from build123d import *

# Parameters (mm, degrees)
SKETCH1_R           = 15.875
SKETCH1_R_2         = 1.5875
BOSS_EXTRUDE1_DEPTH = 6.35
BOSS_EXTRUDE2_START = -6.35
SKETCH2_R           = 1.5875
BOSS_EXTRUDE2_DEPTH = 6.35


with BuildPart() as part:
    # Sketch1 → Boss-Extrude1 (new body)
    with BuildSketch(Plane.XY):
        with BuildLine():
            Line((0, -31.75), (76.2, -31.75))
            Line((76.2, -31.75), (76.2, -6.35))
            Line((76.2, -6.35), (31.108519733, -6.35))
            ThreePointArc((31.108519733, -6.35), (-20.080463142, 24.593444248), (0, -31.75))
        make_face()
        Circle(SKETCH1_R, mode=Mode.SUBTRACT)
        with Locations((-25.4, 0)):
            Circle(SKETCH1_R_2, mode=Mode.SUBTRACT)
        with Locations((25.4, 0)):
            Circle(SKETCH1_R_2, mode=Mode.SUBTRACT)
        with Locations((38.1, -19.05)):
            Circle(SKETCH1_R_2, mode=Mode.SUBTRACT)
        with Locations((63.5, -19.05)):
            Circle(SKETCH1_R_2, mode=Mode.SUBTRACT)
    extrude(amount=BOSS_EXTRUDE1_DEPTH)

    # Sketch2 → Boss-Extrude2 (add)
    with BuildSketch(Plane.XY.offset(6.35).offset(BOSS_EXTRUDE2_START)):
        with BuildLine():
            Line((76.2, -6.35), (76.2, 19.05))
            Line((76.2, 19.05), (25.4, 19.05))
            ThreePointArc((25.4, 19.05), (30.977301377, 6.961989614), (31.108519733, -6.35))
            Line((31.108519733, -6.35), (76.2, -6.35))
        make_face()
        with Locations((63.5, 6.35)):
            Circle(SKETCH2_R, mode=Mode.SUBTRACT)
    extrude(amount=BOSS_EXTRUDE2_DEPTH)


solid = part.part
Work out the finished part from the listing and answer in its coordinate system (mm). A direction names the side the tool comes from. Give positions to 0.01 mm unless a question says otherwise; leave off trailing zeros. Loops run counter-clockwise (first coordinate to the right, second up) from the corner with the lowest first, then second, coordinate; pieces in that order, holes last. Notation, with made-up numbers: (17.5, 45) - (38.5, 45) arc R10 ccw to (38.5, 50) - close; hole circle Ø7 at (80.5, 19.25). An arc over 180 degrees is marked (long way). Answer in a Markdown table with one row per item.
(1) For a pull along Y with two mould halves and no side action, classify faces 1 (the face through (-26.986, 0.07, 3.131)), 2 (the face through (38, -31.75, 3)), 3 (the face through (64.35, -17.71, 3.13)), 4 (the face through (76.2, -7, 3)) as pulls with the +Y half, pulls with the -Y half, needs draft (parallel to the pull), parting line crosses it, or undercut.
Results list:
| item | result |
|---|---|
| face 1 | undercut |
| face 2 | pulls with the -Y half |
| face 3 | undercut |
| face 4 | needs draft |
(2) Section A-A (x = 38.1) is taken. Give the vertices of the cut face in (y, z).
Results list:
| item | result |
|---|---|
| outline | (-31.75, 0) - (-20.64, 0) - (-20.64, 6.35) - (-31.75, 6.35) - close; (-17.46, 0) - (19.05, 0) - (19.05, 6.35) - (-17.46, 6.35) - close |
(3) Flat-ended cylindrical pins translate along their axes: pin 1 Ø8 at (x, y) = (24.5, 5.5) entering from -Z; pin 2 Ø1.9 at (x, y) = (25.4, 0) entering from -Z; pin 3 Ø2 at (y, z) = (-6.5, 2) entering from -X; pin 4 Ø3 at (x, z) = (-20, 4) entering from +Y. Find the tip coordinate at first contact, or state that the pin passes through.
Results list:
| item | result |
|---|---|
| pin 1 | stops at z = 0 |
| pin 2 | passes through |
| pin 3 | stops at x = -31.27 |
| pin 4 | stops at y = 25.8 |
(4) A tool of negligible diameter and unlimited length cuts with its end or side. For faces 5 (the face through (51, 19.05, 3)), 6 (the face through (26.914, 0.477, 3.131)), from which of +Z, -Z, +X, -X, +Y, -Y can it reach the whole face along a straight path? Write none if from no direction.
Results list:
| item | result |
|---|---|
| face 5 | +Z, -Z, +X, +Y |
| face 6 | +Z, -Z |
(5) Section D-D (x = 63.5) is taken. Give the vertices of the cut face in (y, z), and give its area (3 significant figures).
Results list:
| item | result |
|---|---|
| outline | (-31.75, 0) - (-20.64, 0) - (-20.64, 6.35) - (-31.75, 6.35) - close; (-17.46, 0) - (4.76, 0) - (4.76, 6.35) - (-17.46, 6.35) - close; (7.94, 0) - (19.05, 0) - (19.05, 6.35) - (7.94, 6.35) - close |
| area | 282 mm² |
(6) Consider L1, parallel to Y at x = 63.5, z = 4.75; L2, parallel to Y at x = 0, z = 2.25 (3 decimals); L3, parallel to X at y = -1, z = 5.75. Determine where each line is inside the solid, lowest interval first. Write a range as [from, to].
Results list:
| item | result |
|---|---|
| L1 | y = [-31.75, -20.64], [-17.46, 4.76], [7.94, 19.05] |
| L2 | y = [-31.75, -15.875], [15.875, 31.75] |
| L3 | x = [-31.73, -26.63], [-24.17, -15.84], [15.84, 24.17], [26.63, 76.2] |
(7) Section B-B (z = 3) is taken. State how many separate pieces and enclosed holes the cut face has, and give its area (3 significant figures).
Results list:
| item | result |
|---|---|
| separate pieces | 1 |
| enclosed holes | 6 |
| area | 4,850 mm² |
